from build123d import *

# Parameters (mm, degrees)
SKETCH_W        = 72
SKETCH_H        = 72
PAD_DEPTH       = 1.5
PAD001_DEPTH    = 6
SKETCH002_R     = 1.6
POCKET_DEPTH    = 7.501
FILLET_R        = 2
CHAMFER_SIZE    = 1
POCKET001_DEPTH = 5


with BuildPart() as part:
    # Sketch → Pad (new body)
    with BuildSketch(Plane.XY):
        with Locations((36, -36)):
            Rectangle(SKETCH_W, SKETCH_H)
    extrude(amount=PAD_DEPTH)

    # Sketch001 (on Face6 of Pad) → Pad001 (join)
    with BuildSketch(Plane.XY.offset(1.5)):
        with BuildLine():
            ThreePointArc((0, -8), (5.656854, -5.656854), (8, 0))
            Line((0, 0), (8, 0))
            Line((0, -8), (0, 0))
        make_face()
        with BuildLine():
            ThreePointArc((8, -72), (5.656854, -66.343146), (0, -64))
            Line((0, -72), (0, -64))
            Line((8, -72), (0, -72))
        make_face()
        with BuildLine():
            ThreePointArc((72, -64), (66.343146, -66.343146), (64, -72))
            Line((64, -72), (72, -72))
            Line((72, -72), (72, -64))
        make_face()
        with BuildLine():
            ThreePointArc((64, 0), (66.343146, -5.656854), (72, -8))
            Line((72, -8), (72, 0))
            Line((72, 0), (64, 0))
        make_face()
    extrude(amount=PAD001_DEPTH)

    # Sketch002 (on Face14 of Pad001) → Pocket (cut, through all)
    with BuildSketch(Plane.XY.offset(7.5)):
        with Locations((4, -4)):
            Circle(SKETCH002_R)
        with Locations((68, -4)):
            Circle(SKETCH002_R)
        with Locations((68, -68)):
            Circle(SKETCH002_R)
        with Locations((4, -68)):
            Circle(SKETCH002_R)
    extrude(amount=-POCKET_DEPTH, mode=Mode.SUBTRACT)

    # Fillet
    fillet_edges = [part.edges().sort_by_distance(p)[0] for p in [
        (0, 0, 4.5),
        (72, 0, 4.5),
        (0, -72, 4.5),
        (72, -72, 4.5),
    ]]
    fillet(fillet_edges, radius=FILLET_R)

    # Chamfer
    chamfer_edges = [part.edges().sort_by_distance(p)[0] for p in [
        (36, -72, 0),
    ]]
    chamfer(chamfer_edges, length=CHAMFER_SIZE)

    # Sketch003 (on Face11 of Chamfer) → Pocket001 (cut)
    with BuildSketch(Plane(origin=(0, 0, 0), x_dir=(1, 0, 0), z_dir=(0, 0, -1))):
        with BuildLine():
            ThreePointArc((11, 3), (11.146447, 2.646447), (11.5, 2.5))
            Line((11.5, 2.5), (35.5, 2.5))
            ThreePointArc((35.5, 2.5), (35.853553, 2.646447), (36, 3))
            Line((36, 58), (36, 3))
            ThreePointArc((36, 58), (35.853553, 58.353553), (35.5, 58.5))
            Line((11.5, 58.5), (35.5, 58.5))
            ThreePointArc((11.5, 58.5), (11.146447, 58.353553), (11, 58))
            Line((11, 3), (11, 58))
        make_face()
    extrude(amount=-POCKET001_DEPTH, mode=Mode.SUBTRACT)


solid = part.part
Could you check a few things on this model? Use its own coordinates, in mm. A direction names the side the tool comes from. Give positions to 0.01 mm unless a question says otherwise; leave off trailing zeros. Order: outer loops, then holes, each group sorted by start corner. A loop starts at its lowest first (then second) coordinate and runs counter-clockwise, first axis right, second up. Notation, with made-up numbers: (52.5, 23.25) - (109.5, 23.25) arc R16 cw to (109.5, 45.25) - close; hole circle Ø6 at (67, 79). An arc over 180 degrees is marked (long way). One line per question, with ' | ' between items. Start each with the question number.
Item 1: I'm going to push flat-ended pins straight in: pin 1 Ø3 at (x, y) = (42.5, -25) entering from +Z; pin 2 Ø3 at (x, y) = (68, -4) entering from -Z. Where does each tip first touch, or does it pass through?
Item 2: I need wall thicknesses on probe 1 along Y at (x, z) = (29, 1); probe 2 along X at (y, z) = (-43, 1); probe 3 along X at (y, z) = (-68, 2). Which ranges of each line are inside material? Lowest first, please. Write a range as [from, to].
Item 3: I want a section at D-D on x = 4. Write out the boundary of the cut face in (y, z).
Item 4: Thinking about a two-plate mould opening in Y: for faces 1 (the cylindrical face through (5.719, -66.406, 4.458)), 2 (the conical face through (1, -70.98, 0.4)), 3 (the flat face through (30.8, 0, 1.3)), which applies, pulls with the +Y half, pulls with the -Y half, needs draft (parallel to the pull), parting line crosses it, or undercut?
Item 5: I want a section at C-C on y = -42. Write out the boundary of the cut face in (x, z).
Item 6: I want a section at A-A on z = 2.5. Write out the boundary of the cut face in (x, y), then the cut area to 3 significant figures.
Item 7: I want a section at B-B on x = 19.5. Write out the boundary of the cut face in (y, z).
Item 8: For faces 4 (the cylindrical face through (4.86, -2.65, 3.8)), 5 (the flat face through (43, -43, 1.5)), which set-ups out of +Z, -Z, +X, -X, +Y, -Y let a thin tool reach every point of the face, with its end or its side?
Verdict:
1) pin 1: z = 1.5 | pin 2: through
2) probe 1: [-72, -58.5], [-2.5, 0] | probe 2: [0, 11], [36, 72] | probe 3: [0, 2.4], [5.6, 6.93], [65.07, 66.4], [69.6, 72]
3) outline: (-72, 1) - (-71, 0) - (-69.6, 0) - (-69.6, 7.5) - (-72, 7.5) - close; (-66.4, 0) - (-5.6, 0) - (-5.6, 7.5) - (-6.93, 7.5) - (-6.93, 1.5) - (-65.07, 1.5) - (-65.07, 7.5) - (-66.4, 7.5) - close; (-2.4, 0) - (-1, 0) - (0, 1) - (0, 7.5) - (-2.4, 7.5) - close
4) face 1: undercut | face 2: pulls with the -Y half | face 3: pulls with the +Y half
5) outline: (0, 1) - (1, 0) - (11, 0) - (11, 1.5) - (0, 1.5) - close; (36, 0) - (71, 0) - (72, 1) - (72, 1.5) - (36, 1.5) - close
6) outline: (0, -70) arc R2 ccw to (2, -72) - (8, -72) arc R8 ccw to (0, -64) - close; (0, -8) arc R8 ccw to (8, 0) - (2, 0) arc R2 ccw to (0, -2) - close; (64, -72) - (70, -72) arc R2 ccw to (72, -70) - (72, -64) arc R8 ccw to start; (64, 0) arc R8 ccw to (72, -8) - (72, -2) arc R2 ccw to (70, 0) - close; hole circle Ø3.2 at (4, -68); hole circle Ø3.2 at (4, -4); hole circle Ø3.2 at (68, -68); hole circle Ø3.2 at (68, -4) | area: 165 mm^2
7) outline: (-72, 1) - (-71, 0) - (-58.5, 0) - (-58.5, 1.5) - (-72, 1.5) - close; (-2.5, 0) - (-1, 0) - (0, 1) - (0, 1.5) - (-2.5, 1.5) - close
8) face 4: +Z, -Z | face 5: +Z
